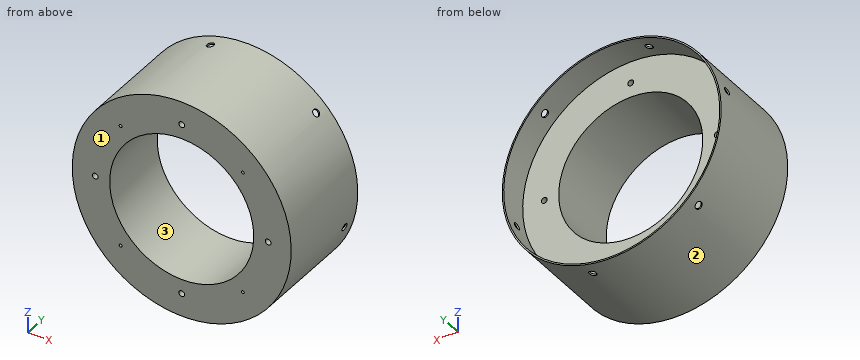
```python
from build123d import *

# Parameters (mm, degrees)
SKETCH_1_R               = 76
EXTRUDE_1_DEPTH          = 70
SKETCH_2_R               = 75
CUT_EXTRUDE_1_DEPTH      = 20
SKETCH_3_R               = 50
CUT_EXTRUDE_3_DEPTH      = 50
SKETCH_4_R               = 2
CUT_EXTRUDE_6_DEPTH      = 70
SKETCH_5_R               = 1
CUT_EXTRUDE_7_DEPTH      = 10
PATTERN_CIRCULAR_1_COUNT = 4
PATTERN_CIRCULAR_2_COUNT = 6


with BuildPart() as part:
    # 草圖1 → 填料-伸長1 (new body)
    with BuildSketch(Plane(origin=(0, 0, 0), x_dir=(1, 0, 0), z_dir=(0, 1, 0))):
        with Locations(Location((0, 0, 0), (0, 0, 270))):
            Circle(SKETCH_1_R)
    extrude(amount=EXTRUDE_1_DEPTH)

    # 草圖2 → 除料-伸長1 (cut)
    with BuildSketch(Plane(origin=(0, 70, 0), x_dir=(1, 0, 0), z_dir=(0, 1, 0))):
        with Locations(Location((0, 0, 0), (0, 0, 270))):
            Circle(SKETCH_2_R)
    extrude(amount=-CUT_EXTRUDE_1_DEPTH, mode=Mode.SUBTRACT)

    # 草圖3 → 除料-伸長3 (cut)
    with BuildSketch(Plane(origin=(0, 50, 0), x_dir=(1, 0, 0), z_dir=(0, 1, 0))):
        with Locations(Location((0, 0, 0), (0, 0, 270))):
            Circle(SKETCH_3_R)
    extrude(amount=-CUT_EXTRUDE_3_DEPTH, mode=Mode.SUBTRACT)

    # 草圖4 → 除料-伸長6 (cut)
    with BuildSketch(Plane.XZ):
        with Locations(Location((-60, 0, 0), (0, 0, 270))):
            Circle(SKETCH_4_R)
        with Locations(Location((0, 60, 0), (0, 0, 270))):
            Circle(SKETCH_4_R)
        with Locations(Location((60, 0, 0), (0, 0, 270))):
            Circle(SKETCH_4_R)
        with Locations(Location((0, -60, 0), (0, 0, 270))):
            Circle(SKETCH_4_R)
    extrude(amount=-CUT_EXTRUDE_6_DEPTH, mode=Mode.SUBTRACT)

    # 草圖5 → 除料-伸長7 (cut)
    with BuildSketch(Plane(origin=(0, 0, 0), x_dir=(-1, 0, 0), z_dir=(0, -1, 0))):
        with Locations(Location((-42.426406871, 42.426406871, 0), (0, 0, 90))):
            Circle(SKETCH_5_R)
    cut_extrude_7 = extrude(amount=-CUT_EXTRUDE_7_DEPTH, mode=Mode.SUBTRACT)

    # 環狀複製排列1: 除料-伸長7 ×4 about axis
    pattern_circular_1_axis = Axis((0, 0, 0), (0, 1, 0))
    for i in range(1, PATTERN_CIRCULAR_1_COUNT):
        add(cut_extrude_7.rotate(pattern_circular_1_axis, i * 360 / PATTERN_CIRCULAR_1_COUNT), mode=Mode.SUBTRACT)

    # 草圖7 → M6  螺絲攻的螺孔鑽1 (revolve, cut)
    with BuildSketch(Plane(origin=(53.740115, 60, 53.74011574), x_dir=(0.7071067860573056, 0, -0.7071067763157894), z_dir=(0, 1, 0))):
        Polygon((0, 0), (0, 36.502151548), (2.5, 35), (2.5, 0), align=None)
    hole_wizard_m6_1 = revolve(axis=Axis((58.23024303, 60, 58.230243832), (-0.7071067763157894, 0, -0.7071067860573056)), mode=Mode.SUBTRACT)

    # 環狀複製排列2: M6  螺絲攻的螺孔鑽1 ×6 about axis
    pattern_circular_2_axis = Axis((0, 70, 0), (0, 1, 0))
    for i in range(1, PATTERN_CIRCULAR_2_COUNT):
        add(hole_wizard_m6_1.rotate(pattern_circular_2_axis, i * 360 / PATTERN_CIRCULAR_2_COUNT), mode=Mode.SUBTRACT)


solid = part.part
```
The model under review builds one solid part; all positions refer to its coordinate system, in mm. Face numbers are marked on the shaded views. Round coordinates to 2 decimals unless told otherwise and drop trailing zeros. Loops run counter-clockwise (first coordinate to the right, second up) from the corner with the lowest first, then second, coordinate; pieces in that order, holes last. Notation, with made-up numbers: M 22.5,59.5 L 68.5,59.5 A15 cw 68.5,70.5 Z; hole C -35,66.25 d4. An arc over 180 degrees is marked long. Write item = value, one per line.
Item 1: Insertion check: P1, Ø5, axis at x = 0, z = 60, coming from the +Y side; P2, Ø4, axis at y = 30.5, z = 58.5, coming from the -X side; P3, Ø1.5, axis at y = 32.5, z = 27, coming from the -X side; P4, Ø1.6, axis at x = -42.5, z = 42, coming from the -Y side. Each pin has a flat end and moves straight along its axis. Give the tip position at first contact, or say it passes through.
Return value:
P1 = 50
P2 = -50.83
P3 = -71.32
P4 = 0
Item 2: Take a section at A-A on x = 0. Write out the cut boundary in (y, z).
Return value:
outline = M 0,-76 L 70,-76 L 70,-75 L 50,-75 L 50,-62 L 0,-62 Z; M 0,-58 L 50,-58 L 50,-50 L 0,-50 Z; M 0,50 L 50,50 L 50,58 L 0,58 Z; M 0,62 L 50,62 L 50,75 L 70,75 L 70,76 L 0,76 Z
Item 3: For line 1 (X direction, y = 20, z = 0); line 2 (X direction, y = 59, z = 0); line 3 (Z direction, x = 19.5, y = 36), list the stretches that pass through material, from the lowest coordinate up. Write a range as [from, to].
Return value:
line_1 = [-76, -62], [-58, -50], [50, 58], [62, 76]
line_2 = [-76, -75], [75, 76]
line_3 = [-73.46, -46.04], [46.04, 73.46]
Item 4: Take a section at C-C on z = 0. Write out the cut boundary in (x, y), then the cut area to 3 significant figures.
Return value:
outline = M -76,0 L -62,0 L -62,50 L -75,50 L -75,70 L -76,70 Z; M -58,0 L -50,0 L -50,50 L -58,50 Z; M 50,0 L 58,0 L 58,50 L 50,50 Z; M 62,0 L 76,0 L 76,70 L 75,70 L 75,50 L 62,50 Z
area = 2,240 mm2
Item 5: Take a section at D-D on x = 60. Write out the cut boundary in (y, z).
Return value:
outline = M 0,-46.65 L 70,-46.65 L 70,-45 L 50,-45 L 50,-2 L 0,-2 Z; M 0,2 L 50,2 L 50,45 L 70,45 L 70,46.65 L 0,46.65 Z
Item 6: The part is to be moulded in two halves that separate along Z. For the marked faces 1, 2 and 3, say which applies: released by +Z, released by -Z, zero draft, split by the parting line, or undercut.
Return value:
face_1 = zero draft
face_2 = split by the parting line
face_3 = undercut
Item 7: Take a section at B-B on y = 43. Write out the cut boundary in (x, z).
Return value:
outline = C 0,0 d152; hole C -60,0 d4; hole C 0,0 d100; hole C 0,-60 d4; hole C 0,60 d4; hole C 60,0 d4
